```python
from build123d import *

# Parameters (mm, degrees)
F0_W     = 5
F0_H     = 5
F1_DEPTH = 0.1
F2_DEPTH = 0.5
F3_DEPTH = 0.7
F4_DEPTH = 1
F5_DEPTH = 1.5
F6_DEPTH = 2
F7_DEPTH = 0.2
F8_DEPTH = 0.3


with BuildPart() as f1:
    # F0 (on Top) → F1 (new body)
    with BuildSketch(Plane.XY):
        with Locations((-17.5, 0)):
            Rectangle(F0_W, F0_H)
    extrude(amount=F1_DEPTH)

    # F0 (on Top) → F7 (join)
    with BuildSketch(Plane.XY):
        with Locations((-12.5, 0)):
            Rectangle(F0_W, F0_H)
    extrude(amount=F7_DEPTH)



with BuildPart() as f2:
    # F0 (on Top) → F2 (new body)
    with BuildSketch(Plane.XY):
        with Locations((-2.5, 0)):
            Rectangle(F0_W, F0_H)
    extrude(amount=F2_DEPTH)

    # F0 (on Top) → F3 (join)
    with BuildSketch(Plane.XY):
        with Locations((2.5, 0)):
            Rectangle(F0_W, F0_H)
    extrude(amount=F3_DEPTH)

    # F0 (on Top) → F4 (join)
    with BuildSketch(Plane.XY):
        with Locations((7.5, 0)):
            Rectangle(F0_W, F0_H)
    extrude(amount=F4_DEPTH)

    # F0 (on Top) → F5 (join)
    with BuildSketch(Plane.XY):
        with Locations((12.5, 0)):
            Rectangle(F0_W, F0_H)
    extrude(amount=F5_DEPTH)

    # F0 (on Top) → F6 (join)
    with BuildSketch(Plane.XY):
        with Locations((17.5, 0)):
            Rectangle(F0_W, F0_H)
    extrude(amount=F6_DEPTH)


with BuildPart() as f1_1:
    add(f1.part)

    add(f2.part)  # F8 merges F2
    # F0 (on Top) → F8 (join)
    with BuildSketch(Plane.XY):
        with Locations((-7.5, 0)):
            Rectangle(F0_W, F0_H)
    extrude(amount=F8_DEPTH)


solid = f1_1.part
```
Geometry: final body of the model. Coordinates: model frame, mm. A direction names the side the tool comes from. Round coordinates to 2 decimals unless told otherwise and drop trailing zeros. Write each loop counter-clockwise with the first axis right and the second up, starting at its lowest first coordinate (ties: lowest second). Pieces come first, ordered by that corner, then holes.
Item 1: Section query B-B (x = 7). Return loops of the section in (y, z), plus the area to 3 significant figures.
Item 2: Section query A-A (y = 1.4). Return loops of the section in (x, z), plus the area to 3 significant figures.
Item 3: Pin query (flat end, axial travel): P1, Ø1.5, axis at x = -1.5, y = 1, coming from the +Z side; P2, Ø1.5, axis at x = 8, y = 0.5, coming from the +Z side; P3, Ø2.5, axis at x = -13.5, y = 1, coming from the +Z side. Return the tip coordinate at first contact, or that it passes through.
Item 4: Material intervals for L1, parallel to Z at x = 6.5, y = -2; L2, parallel to X at y = -0.5, z = 0.35; L3, parallel to Z at x = -6, y = -0.35, sorted ascending.
Item 5: Section query C-C (x = 11). Return loops of the section in (y, z), plus the area to 3 significant figures.
Item 6: Set-up query: faces 1 (the face through (20, 0, 1)), 2 (the face through (12, 0, 1.5)). Return all of +Z, -Z, +X, -X, +Y, -Y with unobstructed straight access to the full face (end or side cutting, diameter ignored); none if empty.
Completed:
1. outline: (-2.5, 0) - (2.5, 0) - (2.5, 1) - (-2.5, 1) - close
1. area: 5.00 mm2
2. outline: (-20, 0) - (20, 0) - (20, 2) - (15, 2) - (15, 1.5) - (10, 1.5) - (10, 1) - (5, 1) - (5, 0.7) - (0, 0.7) - (0, 0.5) - (-5, 0.5) - (-5, 0.3) - (-10, 0.3) - (-10, 0.2) - (-15, 0.2) - (-15, 0.1) - (-20, 0.1) - close
2. area: 31.5 mm2
3. P1: stops at z = 0.5
3. P2: stops at z = 1
3. P3: stops at z = 0.2
4. L1: z = 0 to 1
4. L2: x = -5 to 20
4. L3: z = 0 to 0.3
5. outline: (-2.5, 0) - (2.5, 0) - (2.5, 1.5) - (-2.5, 1.5) - close
5. area: 7.50 mm2
6. face 1: +Z, -Z, +X, +Y, -Y
6. face 2: +Z, -X, +Y, -Y
